CAD build for the part. Positions are in the model's coordinates, mm. Face numbers are marked on the shaded views. Round coordinates to 2 decimals unless told otherwise and drop trailing zeros. Loops run counter-clockwise (first coordinate to the right, second up) from the corner with the lowest first, then second, coordinate; pieces in that order, holes last.
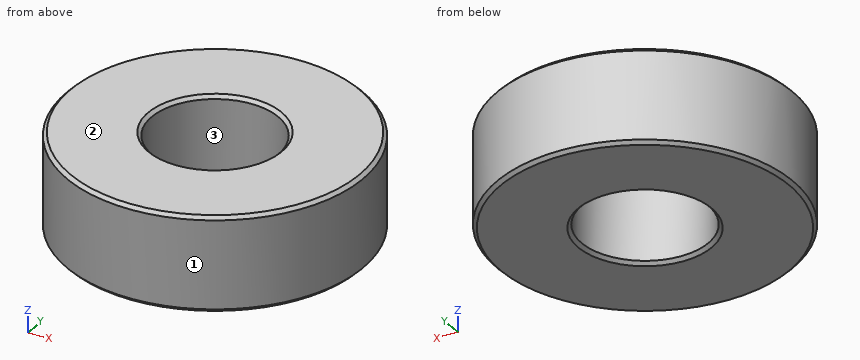
```python
from build123d import *

# Parameters (mm, degrees)
SKETCH1_W     = 6.35
SKETCH1_H     = 7.112
CHAMFER1_SIZE = 0.254


with BuildPart() as part:
    # Sketch1 → Revolve1 (revolve)
    with BuildSketch(Plane(origin=(0, 0, 0), x_dir=(1, 0, 0), z_dir=(0, 1, 0))):
        with Locations((7.9375, -3.556)):
            Rectangle(SKETCH1_W, SKETCH1_H)
    revolve(axis=Axis((0, 0, 0), (0, 0, 1)))

    # Chamfer1
    chamfer1_edges = [part.edges().sort_by_distance(p)[0] for p in [
        (-11.1125, 0, 0),
        (-11.1125, 0, 7.112),
        (-4.7625, 0, 7.112),
        (-4.7625, 0, 0),
    ]]
    chamfer(chamfer1_edges, length=CHAMFER1_SIZE)


solid = part.part
```
Item 1: Two-plate mould, pull along Y, no slides. Class the marked faces 1, 2 and 3: released by +Y, released by -Y, zero draft, split by the parting line, or undercut.
Answers follow:
face 1: split by the parting line
face 2: zero draft
face 3: undercut
Item 2: Cut at C-C, the plane z = 2.5. Give the cut face in (x, y) (1 decimal).
Answers follow:
outline: circle Ø22.2 at (0, 0); hole circle Ø9.5 at (0, 0)
Item 3: Cut at A-A, the plane x = 0. Give the cut face in (y, z), plus the area to 3 significant figures.
Answers follow:
outline: (-11.11, 0.25) - (-10.86, 0) - (-5.02, 0) - (-4.76, 0.25) - (-4.76, 6.86) - (-5.02, 7.11) - (-10.86, 7.11) - (-11.11, 6.86) - close; (4.76, 0.25) - (5.02, 0) - (10.86, 0) - (11.11, 0.25) - (11.11, 6.86) - (10.86, 7.11) - (5.02, 7.11) - (4.76, 6.86) - close
area: 90.1 mm2
Item 4: Probe line 1 (Y direction, x = 0, z = 2); line 2 (X direction, y = 2, z = 3.75); line 3 (Y direction, x = -2.75, z = 5.5). List the from-to ranges inside material, lowest first.
Answers follow:
line 1: y = -11.11 to -4.76, 4.76 to 11.11
line 2: x = -10.93 to -4.32, 4.32 to 10.93
line 3: y = -10.77 to -3.89, 3.89 to 10.77
